The listing builds one solid part. Answer for the finished solid, in the listing's coordinates (mm). Face numbers are marked on the shaded views. A direction names the side the tool comes from. Give positions to 0.01 mm unless a question says otherwise; leave off trailing zeros. Loops run counter-clockwise (first coordinate to the right, second up) from the corner with the lowest first, then second, coordinate; pieces in that order, holes last. Notation, with made-up numbers: M -12,20 L 3,20 A26 ccw 3,48 Z; hole C 27.5,-25 d2. An arc over 180 degrees is marked long. Use one line per item in the form item = value. Start each with the question number.
1. Each of these flat-tipped pins is pushed along its axis until it touches: pin 1 Ø7.5 at (y, z) = (19.5, -12) entering from +X; pin 2 Ø3 at (x, z) = (-4, -13) entering from -Y; pin 3 Ø1.9 at (x, y) = (-0.5, 16.5) entering from -Z. Where does it stop, or does it pass through?
2. The part is cut by section B-B (y = 10). Write down the section's boundary in (x, z) (3 decimals).
3. The part is cut by section D-D (y = 21.5). Write down the section's boundary in (x, z) (3 decimals), and give its area (3 significant figures).
4. The mould has two halves that part along Y. Classify the marked faces 4, 5, 6 and 7: released by +Y, released by -Y, zero draft, split by the parting line, or undercut.
5. The part is cut by section A-A (x = 0). Write down the section's boundary in (y, z), and give its area (3 significant figures).
6. Straight lines are drawn through the part: line 1 (Z direction, x = -1.25, y = 11); line 2 (Z direction, x = 0.5, y = 12.75); line 3 (Y direction, x = -8.75, z = -10.5). For each, find the intervals that lie inside material, in ascending order. Write a range as from..to.
7. The part is cut by section C-C (z = 1.5). Write down the section's boundary in (x, y), and give its area (3 significant figures).
8. For the marked faces 1, 2 and 3, determine the directions among +Z, -Z, +X, -X, +Y, -Y from which every point of the face is accessible in a straight line to the end or side of a thin tool.
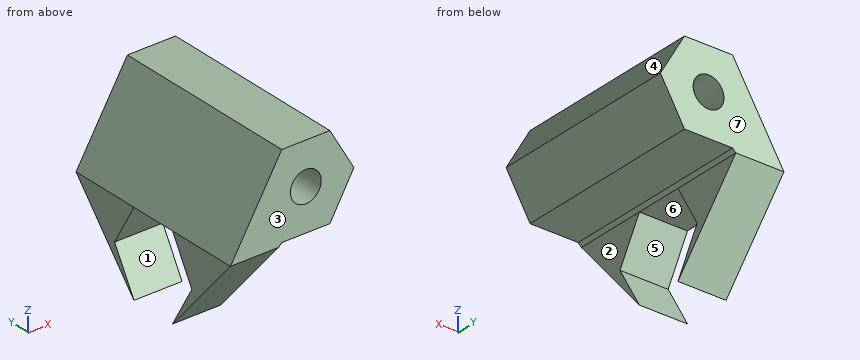
from build123d import *

# Parameters (mm, degrees)
BOSS_EXTRUDE1_DEPTH = 25.4
SKETCH3_R           = 2.032
CUT_EXTRUDE1_DEPTH  = 25.4
BOSS_EXTRUDE2_DEPTH = 25.4
BOSS_EXTRUDE4_DEPTH = 6.35


with BuildPart() as part:
    # Sketch1 → Boss-Extrude1 (new body)
    with BuildSketch(Plane(origin=(0, 0, 0), x_dir=(1, 0, 0), z_dir=(0, 1, 0))):
        Polygon((3.175, 5.499261314), (-3.175, 5.499261314), (-6.35, 0), (-3.175, -5.499261314), (3.175, -5.499261314), (6.35, 0), align=None)
    extrude(amount=BOSS_EXTRUDE1_DEPTH)

    # Sketch3 → Cut-Extrude1 (cut)
    with BuildSketch(Plane(origin=(0, 25.4, 0), x_dir=(1, 0, 0), z_dir=(0, 1, 0))):
        with Locations(Location((0, 0, 0), (0, 0, 270))):
            Circle(SKETCH3_R)
    extrude(amount=-CUT_EXTRUDE1_DEPTH, mode=Mode.SUBTRACT)

    # Sketch2 → Boss-Extrude2 (add)
    with BuildSketch(Plane(origin=(0, 25.4, 0), x_dir=(1, 0, 0), z_dir=(0, 1, 0))):
        Polygon((-3.175, -5.499261314), (-9.950369343, 5.924630657), (-3.600369343, 5.924630657), (-3.175, 5.499261314), (-6.35, 0), align=None)
    extrude(amount=-BOSS_EXTRUDE2_DEPTH)

    # Sketch5 → Boss-Extrude4 (add)
    with BuildSketch(Plane.ZY.offset(9.950369343)):
        Polygon((-5.924630657, 15.875), (-11.423891971, 19.05), (-16.923153285, 15.875), (-5.924630657, 25.4), align=None)
        Polygon((-16.923153285, 9.525), (-5.924630657, 0), (-5.924630657, 9.525), (-11.423891971, 6.35), align=None)
    extrude(amount=-BOSS_EXTRUDE4_DEPTH)


solid = part.part
Derived:
q1.pin_1 = -3.6
q1.pin_2 = 4.83
q1.pin_3 = -5.5
q2.outline = M -9.95,-5.925 L -3.6,-5.925 L -3.175,-5.499 L 3.175,-5.499 L 6.35,0 L 3.175,5.499 L -3.175,5.499 Z; hole C 0,0 d4.064
q3.outline = M -9.95,-10.428 L -3.6,-10.428 L -3.6,-5.925 L -3.175,-5.499 L 3.175,-5.499 L 6.35,0 L 3.175,5.499 L -3.175,5.499 L -9.95,-5.925 Z; hole C 0,0 d4.064
q3.area = 142 mm2
q4.face_4 = zero draft
q4.face_5 = undercut
q4.face_6 = undercut
q4.face_7 = released by +Y
q5.outline = M 0,-5.5 L 25.4,-5.5 L 25.4,-2.03 L 0,-2.03 Z; M 0,2.03 L 25.4,2.03 L 25.4,5.5 L 0,5.5 Z
q5.area = 176 mm2
q6.line_1 = -5.5..-1.6, 1.6..5.5
q6.line_2 = -5.5..-1.97, 1.97..5.5
q6.line_3 = 3.96..6.88, 18.52..21.44
q7.outline = M -5.55,0 L -1.37,0 L -1.37,25.4 L -5.55,25.4 Z; M 1.37,0 L 5.48,0 L 5.48,25.4 L 1.37,25.4 Z
q7.area = 211 mm2
q8.face_1 = +X, -X
q8.face_2 = -Z, +X, +Y, -Y
q8.face_3 = +Z, -Z, +X, -X, -Y
